Source: CAD feature listing. Evaluate the final solid. Frame: model axes, mm. Face numbers are marked on the shaded views. A direction names the side the tool comes from. Coordinates: 2 decimals unless noted, no trailing zeros. Write each loop counter-clockwise with the first axis right and the second up, starting at its lowest first coordinate (ties: lowest second). Pieces come first, ordered by that corner, then holes. Notation, with made-up numbers: M -32.5,38.5 L -4.5,38.5 A13 cw -4.5,59.5 Z; hole C 31.25,-3.75 d4. An arc over 180 degrees is marked long. Answer as CSV lines item,"result". Start each with the question number.
1. Section C-C on x = -104. Return the cut outline in (y, z).
2. Reachability of the marked faces 1 and 2 from +Z, -Z, +X, -X, +Y, -Y: full face, straight path, thin tool, end or side. Return the list, or none.
3. Section D-D on x = -211.5. Return the cut outline in (y, z).
4. Contact query for flat-ended pins moving along their axis: pin 1 Ø2 at (y, z) = (55, 3) entering from -X; pin 2 Ø1 at (y, z) = (27.5, 14.5) entering from +X; pin 3 Ø17 at (x, y) = (-202.94, -86.14) entering from -Z; pin 4 Ø1 at (y, z) = (13, 16.5) entering from -X. Output: stop coordinate, or through.
5. Section A-A on x = -56.5. Return the cut outline in (y, z), plus the area to 3 significant figures.
6. Line query: probe 1 along Z at (x, y) = (35, 48); probe 2 along Y at (x, z) = (-17, 15.5); probe 3 along Y at (x, z) = (-41.5, 1.5). Output: solid intervals per line, ascending. Write a range as [from, to].
7. Section B-B on z = 5.25. Return the cut outline in (x, y), plus the area to 3 significant figures.
```python
from build123d import *

# Parameters (mm, degrees)
BOSS_EXTRUDE2_DEPTH = 25.4
SHELL1_T            = -1.5875
SKETCH4_W           = 47.625
SKETCH4_H           = 22.225
CUT_EXTRUDE1_DEPTH  = 25.4
SKETCH5_R           = 14.2875
CUT_EXTRUDE2_DEPTH  = 268.575466435
CUT_EXTRUDE4_DEPTH  = 25.4


with BuildPart() as part:
    # Sketch3 → Boss-Extrude2 (new body)
    with BuildSketch(Plane.XY):
        Polygon((117.084839529, 87.84302106), (-118.985491202, 87.84302106), (-237.562751028, -92.579381795), (-195.110420945, -120.479913519), (-91.583155779, 37.04302106), (117.084839529, 37.04302106), align=None)
    extrude(amount=BOSS_EXTRUDE2_DEPTH)

    # Shell1
    shell1_openings = [part.faces().sort_by_distance(p)[0] for p in [
        (117.084839529, 62.44302106, 12.7),
    ]]
    offset(amount=SHELL1_T, openings=shell1_openings, kind=Kind.INTERSECTION)

    # Sketch4 → Cut-Extrude1 (cut)
    with BuildSketch(Plane(origin=(-114.151230572, -173.687934254, 0), x_dir=(0.8356757890471017, -0.549223065430162, 0), z_dir=(-0.549223065430162, -0.8356757890471017, 0))):
        with Locations((-122.278707548, 12.7)):
            Rectangle(SKETCH4_W, SKETCH4_H)
    extrude(amount=-CUT_EXTRUDE1_DEPTH, mode=Mode.SUBTRACT)

    # Sketch5 → Cut-Extrude2 (cut, through all)
    with BuildSketch(Plane.XY):
        with Locations((-202.936184524, -86.140134233)):
            Circle(SKETCH5_R)
        with Locations((91.684839529, 62.44302106)):
            Circle(SKETCH5_R)
        with Locations((-105.28432349, 62.44302106)):
            Circle(SKETCH5_R)
    extrude(amount=CUT_EXTRUDE2_DEPTH, mode=Mode.SUBTRACT)

    # Sketch6 → Cut-Extrude4 (cut)
    with BuildSketch(Plane.XY.offset(25.4)):
        with BuildLine():
            Line((117.084839529, 81.49302106), (117.084839529, 87.84302106))
            Line((117.084839529, 87.84302106), (110.734839529, 87.84302106))
            ThreePointArc((110.734839529, 87.84302106), (114.135479832, 84.893661363), (117.084839529, 81.49302106))
        make_face()
        with BuildLine():
            Line((117.084839529, 37.04302106), (117.084839529, 43.39302106))
            ThreePointArc((117.084839529, 43.39302106), (114.135479832, 39.992380757), (110.734839529, 37.04302106))
            Line((110.734839529, 37.04302106), (117.084839529, 37.04302106))
        make_face()
        with BuildLine():
            ThreePointArc((-233.314578978, -95.371366566), (-234.181501959, -91.778630344), (-234.625048962, -88.109492152))
            Line((-234.625048962, -88.109492152), (-237.562751028, -92.579381795))
            Line((-237.562751028, -92.579381795), (-233.314578978, -95.371366566))
        make_face()
        with BuildLine():
            Line((-195.110420945, -120.479913519), (-192.172718878, -116.010023876))
            ThreePointArc((-192.172718878, -116.010023876), (-195.716744004, -117.058448847), (-199.358592995, -117.687928749))
            Line((-199.358592995, -117.687928749), (-195.110420945, -120.479913519))
        make_face()
    extrude(amount=-CUT_EXTRUDE4_DEPTH, mode=Mode.SUBTRACT)


solid = part.part
```
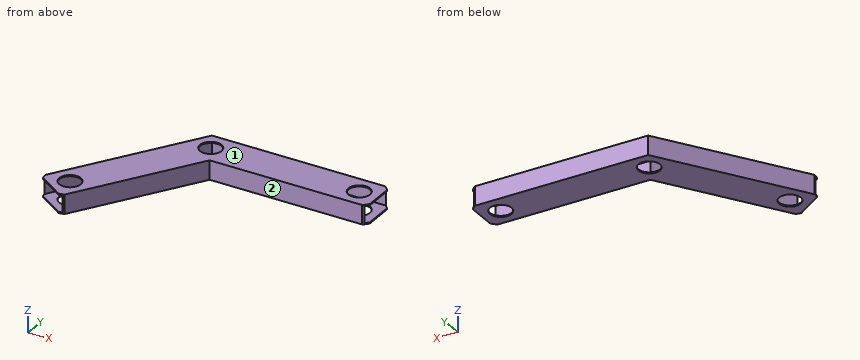
Values:
1,outline,"M 18.15,0 L 48.21,0 L 48.21,1.59 L 21.04,1.59 L 21.04,23.81 L 48.21,23.81 L 48.21,25.4 L 18.15,25.4 Z; M 76.67,0 L 87.84,0 L 87.84,25.4 L 76.67,25.4 L 76.67,23.81 L 86.26,23.81 L 86.26,1.59 L 76.67,1.59 Z"
2,face 1,"+Z, +X, -X, +Y, -Y"
2,face 2,"+Z, -Z, +X, -Y"
3,outline,"M -109.71,0 L -97.58,0 L -97.58,1.59 L -109.71,1.59 Z; M -109.71,23.81 L -97.58,23.81 L -97.58,25.4 L -109.71,25.4 Z; M -74.7,0 L -52.92,0 L -52.92,25.4 L -74.7,25.4 L -74.7,23.81 L -55.81,23.81 L -55.81,1.59 L -74.7,1.59 Z"
4,pin 1,"x = -141.23"
4,pin 2,"x = -97.53"
4,pin 3,"through"
4,pin 4,"x = -168.5"
5,outline,"M 37.04,0 L 87.84,0 L 87.84,25.4 L 37.04,25.4 Z; hole M 38.63,1.59 L 86.26,1.59 L 86.26,23.81 L 38.63,23.81 Z"
5,area,"232 mm²"
6,probe 1,"[0, 1.59], [23.81, 25.4]"
6,probe 2,"[37.04, 38.63], [86.26, 87.84]"
6,probe 3,"[37.04, 87.84]"
7,outline,"M -234.63,-88.11 A31.75 ccw -234.37,-90.61 L -118.13,86.26 L 112.69,86.26 A31.75 ccw 110.73,87.84 L -118.99,87.84 Z; M -194.57,-116.77 A31.75 ccw -192.17,-116.01 L -91.58,37.04 L 110.73,37.04 A31.75 ccw 112.69,38.63 L -92.44,38.63 Z"
7,area,"1,320 mm²"
